Source: CAD feature listing. Evaluate the final solid. Frame: model axes, mm. Face numbers are marked on the shaded views. A direction names the side the tool comes from. Give positions to 0.01 mm unless a question says otherwise; leave off trailing zeros. Loops run counter-clockwise (first coordinate to the right, second up) from the corner with the lowest first, then second, coordinate; pieces in that order, holes last. Notation, with made-up numbers: M 45.25,18 L 74.25,18 A22 cw 74.25,44 Z; hole C -24.5,85.5 d5. An arc over 180 degrees is marked long. Put each result on its own line as item: value.
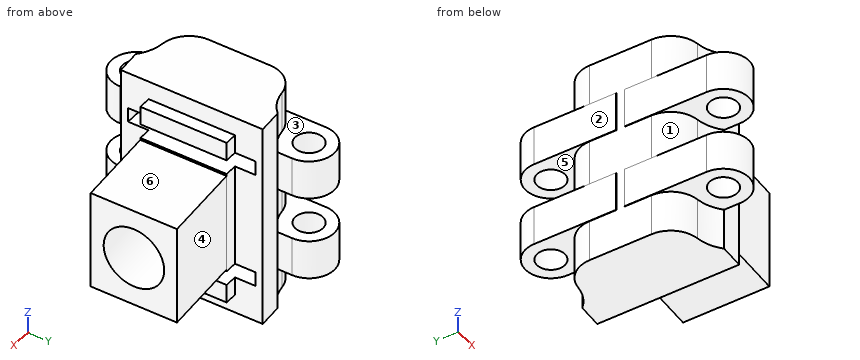
from build123d import *

# Parameters (mm, degrees)
SKETCH4_W               = 13
SKETCH4_H               = 29
BOSS_EXTRUDE1_DEPTH     = 50
SKETCH6_R               = 3.35
BOSS_EXTRUDE2_DEPTH     = 4.75
MIRROR2_COPY_1_SKETCH_R = 3.35
MIRROR2_COPY_1_DEPTH    = 4.75
FILLET2_R               = 7
SKETCH7_W               = 50
SKETCH7_H               = 34.11
BOSS_EXTRUDE3_DEPTH     = 6
BOSS_EXTRUDE4_REACH     = 60.145
CUT_EXTRUDE1_DEPTH      = 59.144819202
SKETCH10_W              = 41
SKETCH10_H              = 21
BOSS_EXTRUDE5_DEPTH     = 3
FILLET4_R               = 10
CUT_EXTRUDE2_DEPTH      = 60.713063897
CUT_EXTRUDE2_DEPTH_BACK = 7
SKETCH11_W              = 3.5
SKETCH11_H              = 31
SKETCH12_W              = 24
SKETCH12_H              = 21
BOSS_EXTRUDE7_DEPTH     = 20
SKETCH15_R              = 7.35
CUT_EXTRUDE3_DEPTH      = 24


with BuildPart() as part:
    # Sketch4 → Boss-Extrude1 (new body)
    with BuildSketch(Plane.XY):
        with Locations((0.5, 0)):
            Rectangle(SKETCH4_W, SKETCH4_H)
    extrude(amount=BOSS_EXTRUDE1_DEPTH)

    # Sketch6 → Boss-Extrude2 (add, symmetric)
    with BuildSketch(Plane.XY.offset(14.75)):
        with BuildLine():
            Line((6.1, 1), (6.1, 21))
            ThreePointArc((6.1, 21), (0, 27.1), (-6.1, 21))
            Line((-6.1, 21), (-6.1, 1))
            Line((-6.1, 1), (6.1, 1))
        make_face()
        with Locations((0, 21)):
            Circle(SKETCH6_R, mode=Mode.SUBTRACT)
    boss_extrude2 = extrude(amount=BOSS_EXTRUDE2_DEPTH, both=True)

    # Mirror1: Boss-Extrude2 across plane
    add(boss_extrude2.mirror(Plane.XY.offset(25)))

    # Mirror2: Boss-Extrude2 across plane
    add(boss_extrude2.mirror(Plane.ZX))

    # Mirror2 copy 1 sketch → Mirror2 copy 1 (add, symmetric)
    with BuildSketch(Plane(origin=(0, 0, 35.25), x_dir=(1, 0, 0), z_dir=(0, 0, -1))):
        with BuildLine():
            Line((6.1, 1), (6.1, 21))
            ThreePointArc((6.1, 21), (0, 27.1), (-6.1, 21))
            Line((-6.1, 21), (-6.1, 1))
            Line((-6.1, 1), (6.1, 1))
        make_face()
        with Locations((0, 21)):
            Circle(MIRROR2_COPY_1_SKETCH_R, mode=Mode.SUBTRACT)
    extrude(amount=MIRROR2_COPY_1_DEPTH, both=True)

    # Fillet2
    fillet2_edges = [part.edges().sort_by_distance(p)[0] for p in [
        (-6, 14.5, 5),
        (-6, 14.5, 25),
        (-6, -14.5, 5),
        (-6, -14.5, 25),
        (-6, 14.5, 45),
        (-6, -14.5, 45),
    ]]
    fillet(fillet2_edges, radius=FILLET2_R)

    # Sketch7 → Boss-Extrude3 (add)
    with BuildSketch(Plane(origin=(6.1, 0, 0), x_dir=(0, 0, -1), z_dir=(1, 0, 0))):
        with Locations((-25, 0)):
            Rectangle(SKETCH7_W, SKETCH7_H)
    extrude(amount=BOSS_EXTRUDE3_DEPTH)

    # Boss-Extrude4: up to this face of the body (flat: up to its plane)
    boss_extrude4_end = Plane(part.part.faces().sort_by_distance((3.691573852, 0, 0))[0])
    # Sketch8 → Boss-Extrude4 (add, up to the picked face)
    with BuildSketch(Plane.XY.offset(50), mode=Mode.PRIVATE) as boss_extrude4_sk1:
        Polygon((6.1, 17.481553553), (12.1, 17.901114425), (12.1, 17.055), (6.1, 17.055), align=None)
    boss_extrude4_tool1 = split(extrude(boss_extrude4_sk1.sketch, amount=-BOSS_EXTRUDE4_REACH, mode=Mode.PRIVATE), bisect_by=boss_extrude4_end, keep=Keep.BOTH, mode=Mode.PRIVATE)
    add(boss_extrude4_tool1.solids().sort_by(Axis((9.42967, 17.384693, 50), (0, 0, -1)))[0])

    # Sketch9 → Cut-Extrude1 (cut, through all)
    with BuildSketch(Plane.XY.offset(50)):
        Polygon((6.1, -17.055), (17.728439632, -16.241860289), (17.728439632, -20.144237666), (6.1, -20.144237666), align=None)
    extrude(amount=-CUT_EXTRUDE1_DEPTH, mode=Mode.SUBTRACT)

    # Sketch10 → Boss-Extrude5 (add)
    with BuildSketch(Plane(origin=(12.1, 0, 0), x_dir=(0, 0, -1), z_dir=(1, 0, 0))):
        with Locations((-25, 0.632837648)):
            Rectangle(SKETCH10_W, SKETCH10_H)
    extrude(amount=BOSS_EXTRUDE5_DEPTH)

    # Fillet4
    # the kernel refuses this fillet: 10 mm, written as the material it adds along each edge
    with BuildSketch(Plane(origin=(6.1, -14.5, 50), x_dir=(0, -1, 0), z_dir=(0, 0, -1))) as fillet4_piece_1:
        with BuildLine():
            CenterArc((9.918128411, 6.76641264), FILLET4_R, 185.625410645, 36.956323183)
            Line((-0.033711831, 5.78616991), (-1.028895855, 5.688145638))
            ThreePointArc((-1.028895855, 5.688145638), (-1, 5.1), (-1, 0))
            Line((-1, 0), (0, -1))
            ThreePointArc((0, -1), (1.2775, -1), (1.818687159, -0.676641264))
            Line((1.818687159, -0.676641264), (2.555, 0))
        make_face()
    extrude(amount=24.465670292)
    with BuildSketch(Plane(origin=(6.1, -14.5, 44.965670292), x_dir=(0, -1, 0), z_dir=(0, 0, -1))) as fillet4_piece_2:
        with BuildLine():
            CenterArc((9.918128411, 6.76641264), FILLET4_R, 185.625410645, 36.956323183)
            Line((-0.033711831, 5.78616991), (-1.028895855, 5.688145638))
            ThreePointArc((-1.028895855, 5.688145638), (-1, 5.1), (-1, 0))
            Line((-1, 0), (0, -1))
            ThreePointArc((0, -1), (1.2775, -1), (1.818687159, -0.676641264))
            Line((1.818687159, -0.676641264), (2.555, 0))
        make_face()
    extrude(amount=39.931340584)
    with BuildSketch(Plane(origin=(6.1, -14.5, 24.465670292), x_dir=(-0.9999830276779416, 0.005826178512287368, 0), z_dir=(0, 0, -1))) as fillet4_piece_3:
        with BuildLine():
            CenterArc((6.708513011, -9.957382405), FILLET4_R, 95.291593317, 36.956323183)
            Line((-0.014885886, -2.554956636), (-0.687225776, -1.814714059))
            ThreePointArc((-0.687225776, -1.814714059), (-1.007425971, -1.271652139), (-0.999983028, 0.005826179))
            Line((-0.999983028, 0.005826179), (0.005826179, 0.999983028))
            ThreePointArc((0.005826179, 0.999983028), (5.10573962, 0.970269517), (5.694043627, 0.99573824))
            Line((5.694043627, 0.99573824), (5.786268117, 0))
        make_face()
    extrude(amount=24.465670292)
    with BuildSketch(Plane(origin=(6.1, 14.5, 0), x_dir=(-0.9999554494088081, -0.009439237131707428, 0), z_dir=(0, 0, 1))) as fillet4_piece_4:
        with BuildLine():
            CenterArc((7.162570226, -9.930782909), FILLET4_R, 96.745204553, 39.23266057)
            Line((-0.028143591, -2.981420723), (-0.747214973, -2.286484504))
            ThreePointArc((-0.747214973, -2.286484504), (-1.014027245, -1.481271124), (-0.999955449, 0.009439237))
            Line((-0.999955449, 0.009439237), (0.009439237, 0.999955449))
            ThreePointArc((0.009439237, 0.999955449), (5.109212029, 0.95181534), (5.870573137, 0.993078291))
            Line((5.870573137, 0.993078291), (5.988027418, 0))
        make_face()
    extrude(amount=24.970068545)
    with BuildSketch(Plane(origin=(6.1, 14.5, 4.529931455), x_dir=(0, 1, 0), z_dir=(0, 0, 1))) as fillet4_piece_5:
        with BuildLine():
            CenterArc((9.862731288, 7.255990144), FILLET4_R, 187.286041034, 39.23266057)
            Line((-0.056522411, 5.987760648), (-1.048447781, 5.860937698))
            ThreePointArc((-1.048447781, 5.860937698), (-1, 5.1), (-1, 0))
            Line((-1, 0), (0, -1))
            ThreePointArc((0, -1), (1.490776776, -1), (2.293435779, -0.725599014))
            Line((2.293435779, -0.725599014), (2.981553553, 0))
        make_face()
    extrude(amount=40.940137089)
    with BuildSketch(Plane(origin=(6.1, 14.5, 25.029931455), x_dir=(0, 1, 0), z_dir=(0, 0, 1))) as fillet4_piece_6:
        with BuildLine():
            CenterArc((9.862731288, 7.255990144), FILLET4_R, 187.286041034, 39.23266057)
            Line((-0.056522411, 5.987760648), (-1.048447781, 5.860937698))
            ThreePointArc((-1.048447781, 5.860937698), (-1, 5.1), (-1, 0))
            Line((-1, 0), (0, -1))
            ThreePointArc((0, -1), (1.490776776, -1), (2.293435779, -0.725599014))
            Line((2.293435779, -0.725599014), (2.981553553, 0))
        make_face()
    extrude(amount=24.970068545)

    # Sketch11 → Cut-Extrude2 (cut, two sides: drawn at the far end of the back side and taken through both)
    with BuildSketch(Plane(origin=(12.1, 0, 0), x_dir=(0, 0, -1), z_dir=(1, 0, 0)).offset(-CUT_EXTRUDE2_DEPTH_BACK)):
        with Locations((-10.75, 0.632837648)):
            Rectangle(SKETCH11_W, SKETCH11_H)
        with Locations((-39.25, 0.632837648)):
            Rectangle(SKETCH11_W, SKETCH11_H)
    extrude(amount=CUT_EXTRUDE2_DEPTH + CUT_EXTRUDE2_DEPTH_BACK, mode=Mode.SUBTRACT)

    # Sketch12 → Boss-Extrude7 (add, along a direction that is not the sketch's normal)
    with BuildSketch(Plane(origin=(15.1, 0, 0), x_dir=(0, 0, -1), z_dir=(1, 0, 0))):
        with Locations((-25, 0.632837648)):
            Rectangle(SKETCH12_W, SKETCH12_H)
    extrude(amount=BOSS_EXTRUDE7_DEPTH, dir=(0.9975640502598245, 0.069756473744122, 0))

    # Sketch15 → Cut-Extrude3 (cut)
    with BuildSketch(Plane(origin=(35.752500693, 2.500058392, 0), x_dir=(0, 0, -1), z_dir=(0.9975640502598246, 0.06975647374412185, 0))):
        with Locations(Location((-25, -0.396449194, 0), (0, 0, 90))):
            Circle(SKETCH15_R)
    extrude(amount=-CUT_EXTRUDE3_DEPTH, mode=Mode.SUBTRACT)


solid = part.part
1. Section query A-A (z = 36). Output: boundary loops of the cut face in (x, y) (3 decimals), plus the area to 3 significant figures.
Found:
outline: M -6.1,-21 A6.1 ccw 6.1,-21 L 6.1,-17.055 L 12.1,-16.635 L 12.1,-9.867 L 15.1,-9.867 L 35.051,-8.472 L 35.051,12.528 L 15.1,11.133 L 12.1,11.133 L 12.1,17.901 L 6.1,17.482 L 6.1,21 A6.1 ccw -6.1,21 L -6.1,1 L -6,1 L -6,-1 L -6.1,-1 Z; hole C 0,-21 d6.7; hole C 0,21 d6.7
area: 1,250 mm^2
2. Section query B-B (x = 2). State how many separate pieces and enclosed holes the cut face has, plus the area to 3 significant figures.
Found:
separate pieces: 5
enclosed holes: 0
area: 1,730 mm^2
3. Contact query for flat-ended pins moving along their axis: P1, Ø1.5, axis at x = 13.5, z = 43, coming from the +Y side; P2, Ø1, axis at x = 9, z = 39.5, coming from the +Y side; P3, Ø1.8, axis at y = -2.5, z = 39.5, coming from the +X side. Output: stop coordinate, or through.
Found:
P1: y = 11.13
P2: y = 17.72
P3: x = 5.1
4. Access query for the marked faces 4, 5 and 6. Directions: +Z, -Z, +X, -X, +Y, -Y. A direction counts if a zero-diameter tool reaches every point of the face in a straight line with its end or side. Return the directions, or none.
Found:
face 4: +Z, -Z, +Y
face 5: -X, +Y
face 6: +Z, +X, +Y, -Y
5. Draft query along Z for the marked faces 1, 2 and 3. Return one class per face: pulls with the +Z half, pulls with the -Z half, needs draft (parallel to the pull), parting line crosses it, or undercut.
Found:
face 1: undercut
face 2: needs draft
face 3: pulls with the +Z half
6. Material intervals for line 1 (Y direction, x = 0, z = 14); line 2 (Z direction, x = 11.5, y = -8.5); line 3 (X direction, y = -21, z = 14), sorted ascending. Write a range as from..to.
Found:
line 1: -27.1..-24.35, -17.65..17.65, 24.35..27.1
line 2: 0..9, 12.5..37.5, 41..50
line 3: -6.1..-3.35, 3.35..6.1
